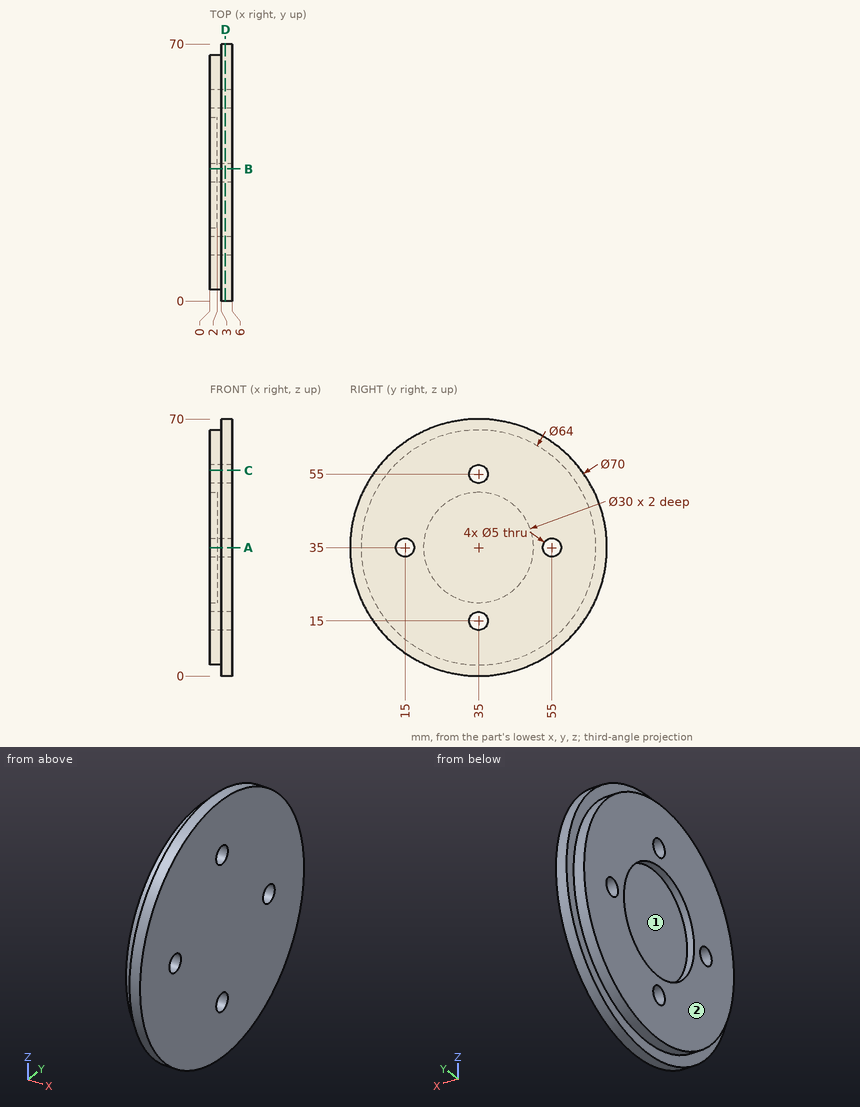
Source: three-view drawing plus pictorial views. Frame: mm from the lowest corner of the part. Round coordinates to 2 decimals unless told otherwise and drop trailing zeros. Loops run counter-clockwise (first coordinate to the right, second up) from the corner with the lowest first, then second, coordinate; pieces in that order, holes last. Notation, with made-up numbers: (-12.75, 1) - (29.25, 1) arc R18 ccw to (29.25, 18) - close; hole circle Ø8 at (-2, 66.25). An arc over 180 degrees is marked (long way). Write each question's results on one line, items separated by ' | '. Start each with the question number.
1) Cut plane C-C on z = 56. Return loops of the section in (x, y), then the cut area to 3 significant figures.
2) Cut plane B-B on y = 36. Return loops of the section in (x, z), then the cut area to 3 significant figures.
3) Mould query, pull axis Z, two halves, no side actions, for the marked faces 1 and 2. Classes: released by +Z, released by -Z, zero draft, split by the parting line, or undercut.
4) Cut plane D-D on x = 4.2. Return loops of the section in (y, z).
5) Line query: probe 1 along Y at (x, z) = (3.6, 35); probe 2 along Y at (x, z) = (4.4, 34.5); probe 3 along X at (y, z) = (6.5, 16.5). Output: solid intervals per line, ascending. Write a range as [from, to].
6) Cut plane A-A on z = 35. Return loops of the section in (x, y).
7) First-contact query: P1, Ø4, axis at y = 15, z = 35, coming from the +X side. Flat tip, straight axial feed; report the tip coordinate or a pass-through.
Verdict:
1) outline: (0, 10.85) - (3, 10.85) - (3, 7) - (6, 7) - (6, 32.71) - (0, 32.71) - close; (0, 37.29) - (6, 37.29) - (6, 63) - (3, 63) - (3, 59.15) - (0, 59.15) - close | area: 285 mm2
2) outline: (0, 3.02) - (3, 3.02) - (3, 0.01) - (6, 0.01) - (6, 12.71) - (0, 12.71) - close; (0, 17.29) - (6, 17.29) - (6, 52.71) - (0, 52.71) - (0, 49.97) - (2, 49.97) - (2, 20.03) - (0, 20.03) - close; (0, 57.29) - (6, 57.29) - (6, 69.99) - (3, 69.99) - (3, 66.98) - (0, 66.98) - close | area: 287 mm2
3) face 1: undercut | face 2: zero draft
4) outline: circle Ø70 at (35, 35); hole circle Ø5 at (15, 35); hole circle Ø5 at (35, 15); hole circle Ø5 at (35, 55); hole circle Ø5 at (55, 35)
5) probe 1: y = [0, 12.5], [17.5, 52.5], [57.5, 70] | probe 2: y = [0, 12.55], [17.45, 52.55], [57.45, 70] | probe 3: x = [3, 6]
6) outline: (0, 3) - (3, 3) - (3, 0) - (6, 0) - (6, 12.5) - (0, 12.5) - close; (0, 17.5) - (6, 17.5) - (6, 52.5) - (0, 52.5) - (0, 50) - (2, 50) - (2, 20) - (0, 20) - close; (0, 57.5) - (6, 57.5) - (6, 70) - (3, 70) - (3, 67) - (0, 67) - close
7) P1: passes through
